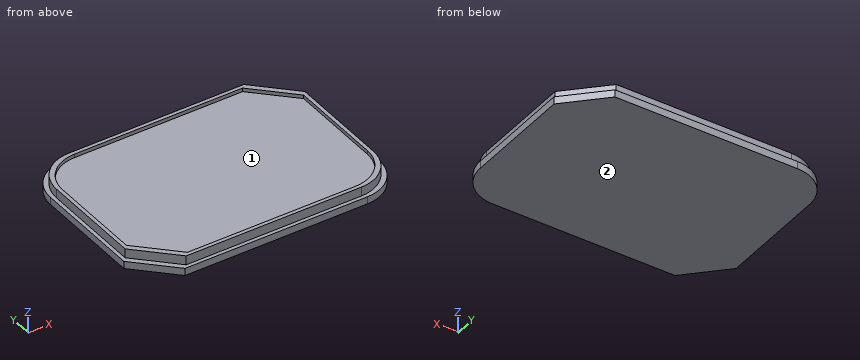
```python
from build123d import *

# Parameters (mm, degrees)
F0_W     = 70
F0_H     = 50
F1_DEPTH = 2
F2_W     = 68
F2_H     = 48
F3_DEPTH = 2.5
F4_W     = 66
F4_H     = 46
F5_DEPTH = 1
F6_SIZE  = 10
F7_R     = 10


with BuildPart() as f1:
    # F0 (on Top) → F1 (new body)
    with BuildSketch(Plane.XY):
        Rectangle(F0_W, F0_H)
    extrude(amount=F1_DEPTH)

    # F2 (on face) → F3 (join)
    with BuildSketch(Plane.XY.offset(2)):
        Rectangle(F2_W, F2_H)
    extrude(amount=F3_DEPTH)

    # F4 (on face) → F5 (cut)
    with BuildSketch(Plane.XY.offset(4.5)):
        Rectangle(F4_W, F4_H)
    extrude(amount=-F5_DEPTH, mode=Mode.SUBTRACT)

    # F6
    f6_edges = [f1.edges().sort_by_distance(p)[0] for p in [
        (33, 23, 4),
        (34, 24, 3.25),
        (35, 25, 1),
        (-33, -23, 4),
        (-34, -24, 3.25),
        (-35, -25, 1),
    ]]
    chamfer(f6_edges, length=F6_SIZE)

    # F7
    f7_edges = [f1.edges().sort_by_distance(p)[0] for p in [
        (33, -23, 4),
        (34, -24, 3.25),
        (35, -25, 1),
        (-33, 23, 4),
        (-34, 24, 3.25),
        (-35, 25, 1),
    ]]
    fillet(f7_edges, radius=F7_R)


solid = f1.part
```
Can you work these out from the model? Positions are in its coordinate system, mm. Face numbers are marked on the shaded views. Coordinates: 2 decimals unless noted, no trailing zeros. Order: outer loops, then holes, each group sorted by start corner. A loop starts at its lowest first (then second) coordinate and runs counter-clockwise, first axis right, second up. Notation, with made-up numbers: (19, -21) -> (61, -21) arc R12 cw to (61, -14) -> close; hole circle Ø11 at (79, -7.5). An arc over 180 degrees is marked (long way). Write each question's results on one line, items separated by ' | '.
Item 1: I want a section at A-A, the plane y = 1.5. Write out the boundary of the cut face in (x, z), then the cut area to 3 significant figures.
Results are:
outline: (-35, 0) -> (35, 0) -> (35, 2) -> (34, 2) -> (34, 4.5) -> (33, 4.5) -> (33, 3.5) -> (-33, 3.5) -> (-33, 4.5) -> (-34, 4.5) -> (-34, 2) -> (-35, 2) -> close | area: 244 mm²
Item 2: I want a section at C-C, the plane x = -2. Write out the boundary of the cut face in (y, z).
Results are:
outline: (-25, 0) -> (25, 0) -> (25, 2) -> (24, 2) -> (24, 4.5) -> (23, 4.5) -> (23, 3.5) -> (-23, 3.5) -> (-23, 4.5) -> (-24, 4.5) -> (-24, 2) -> (-25, 2) -> close
Item 3: I want a section at B-B, the plane z = 0.95. Write out the boundary of the cut face in (x, y).
Results are:
outline: (-35, -15) -> (-25, -25) -> (25, -25) arc R10 ccw to (35, -15) -> (35, 15) -> (25, 25) -> (-25, 25) arc R10 ccw to (-35, 15) -> close
Item 4: If we mould it in two halves opening along Y, with no side actions, what happens to the marked faces 1 and 2? For each: +Y half, -Y half, draft (parallel to the pull), parting line (faces both ways), or undercut.
Results are:
face 1: undercut | face 2: draft
Item 5: If I drill on line 1 along Y through (x, z) = (-4.5, 4.25); line 2 along X through (y, z) = (6, 2.2); line 3 along Z through (x, y) = (3.5, -10), over which ranges is the centre line in solid material (lowest first)?
Results are:
line 1: -24 to -23, 23 to 24 | line 2: -34 to 34 | line 3: 0 to 3.5
Item 6: I'm going to push flat-ended pins straight in: pin 1 Ø3 at (x, y) = (-21.5, -4.5) entering from +Z; pin 2 Ø1.1 at (y, z) = (-2, 4) entering from -X; pin 3 Ø1.2 at (y, z) = (-2, 3.5) entering from +X. Where does each tip first touch, or does it pass through?
Results are:
pin 1: z = 3.5 | pin 2: x = -34 | pin 3: x = 34
